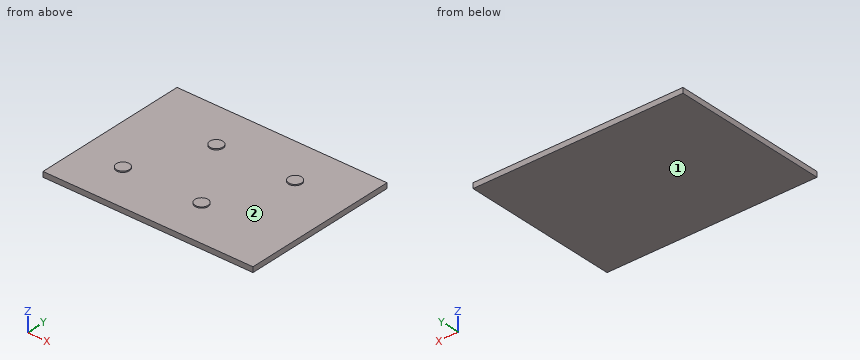
```python
from build123d import *

# Parameters (mm, degrees)
F0_R     = 12.7
F1_DEPTH = 12.446
F0_W     = 406.4
F0_H     = 304.8
F2_DEPTH = 10.16


with BuildPart() as f1:
    # F0 (on Top) → F1 (new body)
    with BuildSketch(Plane.XY):
        with Locations((7.4244239368, 76.3731971383)):
            Circle(F0_R)
    extrude(amount=F1_DEPTH)



with BuildPart() as f1b:
    # F0 (on Top) → F1, piece 2 (new body)
    with BuildSketch(Plane.XY):
        with Locations((159.8244239368, 76.3731971383)):
            Circle(F0_R)
    extrude(amount=F1_DEPTH)


with BuildPart() as f1c:
    # F0 (on Top) → F1, piece 3 (new body)
    with BuildSketch(Plane.XY):
        with Locations((-57.2906026376, -60.2052676494)):
            Circle(F0_R)
    extrude(amount=F1_DEPTH)


with BuildPart() as f1d:
    # F0 (on Top) → F1, piece 4 (new body)
    with BuildSketch(Plane.XY):
        with Locations((95.1093973624, -60.2052676494)):
            Circle(F0_R)
    extrude(amount=F1_DEPTH)


with BuildPart() as f1_1:
    add(f1.part)

    add(f1b.part)  # F2 merges F1b

    add(f1c.part)  # F2 merges F1c

    add(f1d.part)  # F2 merges F1d
    # F0 (on Top) → F2 (join)
    with BuildSketch(Plane.XY):
        with Locations((62.5996744812, 8.4529491862)):
            Rectangle(F0_W, F0_H)
        with Locations((-57.2906026376, -60.2052676494)):
            Circle(F0_R, mode=Mode.SUBTRACT)
        with Locations((95.1093973624, -60.2052676494)):
            Circle(F0_R, mode=Mode.SUBTRACT)
        with Locations((7.4244239368, 76.3731971383)):
            Circle(F0_R, mode=Mode.SUBTRACT)
        with Locations((159.8244239368, 76.3731971383)):
            Circle(F0_R, mode=Mode.SUBTRACT)
    extrude(amount=F2_DEPTH)


solid = f1_1.part
```
The listing builds one solid part. Answer for the finished solid, in the listing's coordinates (mm). Face numbers are marked on the shaded views. A direction names the side the tool comes from. Give positions to 0.01 mm unless a question says otherwise; leave off trailing zeros. Order: outer loops, then holes, each group sorted by start corner. A loop starts at its lowest first (then second) coordinate and runs counter-clockwise, first axis right, second up.
Item 1: The part is cut by section A-A, the plane y = -53. Give the vertices of the cut face in (x, z).
From the geometry:
outline: (-140.6, 0) - (265.8, 0) - (265.8, 10.16) - (105.57, 10.16) - (105.57, 12.45) - (84.65, 12.45) - (84.65, 10.16) - (-46.83, 10.16) - (-46.83, 12.45) - (-67.75, 12.45) - (-67.75, 10.16) - (-140.6, 10.16) - close
Item 2: The part is cut by section B-B, the plane x = -30. Give the vertices of the cut face in (y, z).
From the geometry:
outline: (-143.95, 0) - (160.85, 0) - (160.85, 10.16) - (-143.95, 10.16) - close
Item 3: The part is cut by section D-D, the plane x = 88. Give the vertices of the cut face in (y, z).
From the geometry:
outline: (-143.95, 0) - (160.85, 0) - (160.85, 10.16) - (-49.68, 10.16) - (-49.68, 12.45) - (-70.73, 12.45) - (-70.73, 10.16) - (-143.95, 10.16) - close
Item 4: Which of the six approach directions +Z, -Z, +X, -X, +Y, -Y give full straight-line access (tool end or side, diameter ignored) to the marked faces 1 and 2?
From the geometry:
face 1: -Z, +X, -X, +Y, -Y
face 2: +Z
Item 5: Find the intervals of material crossed by probe 1 along Z at (x, y) = (99, 36); probe 2 along Y at (x, z) = (16, 10.25); probe 3 along Y at (x, z) = (104, 10.5), in increasing order.
From the geometry:
probe 1: z = 0 to 10.16
probe 2: y = 67.01 to 85.74
probe 3: y = -69.27 to -51.14
Item 6: Given pin 1 Ø5 at (x, y) = (126, 17.5) entering from -Z; pin 2 Ø6 at (x, y) = (-35.5, 123) entering from +Z, each flat-ended and moving along its own axis, determine where each tip first touches the part or whether it passes through.
From the geometry:
pin 1: stops at z = 0
pin 2: stops at z = 10.16
Item 7: The part is cut by section C-C, the plane y = 94.5. Give the vertices of the cut face in (x, z), and give its area (3 significant figures).
From the geometry:
outline: (-140.6, 0) - (265.8, 0) - (265.8, 10.16) - (-140.6, 10.16) - close
area: 4,130 mm2
